The model under review builds one solid part; all positions refer to its coordinate system, in mm. Face numbers are marked on the shaded views. A direction names the side the tool comes from. Give positions to 0.01 mm unless a question says otherwise; leave off trailing zeros. Order: outer loops, then holes, each group sorted by start corner. A loop starts at its lowest first (then second) coordinate and runs counter-clockwise, first axis right, second up. Notation, with made-up numbers: M 69,-24 L 88,-24 A9 cw 88,-9 Z; hole C 11.25,65 d5. An arc over 180 degrees is marked long. One line per question, with ' | ' between items. Start each with the question number.
1. We need section C-C on x = -9.65. Write out the cut boundary in (y, z).
2. For the marked faces 1, 2, 3 and 4, list the 3-axis set-ups (+Z, -Z, +X, -X, +Y, -Y) from which the entire face can be reached by the end or side of a thin tool; tool diameter is ignored.
3. Insertion check: P1, Ø5, axis at y = -5.5, z = 6, coming from the +X side; P2, Ø4.5, axis at y = -6.5, z = 4.5, coming from the -X side; P3, Ø5, axis at x = -35, y = -2.5, coming from the +Z side. Each pin has a flat end and moves straight along its axis. Give the tip position at first contact, or say it passes through.
4. We need section D-D on y = -2.5. Count the separate pieces of the cut face and the enclosed holes in it, then the cut area to 3 significant figures.
5. Wall thickness on L1, parallel to X at y = -0.5, z = 5; L2, parallel to X at y = 1.2, z = 0; L3, parallel to X at y = -7.75, z = -6.75: over which ranges is each line inside the solid? List them lowest first.
6. We need section B-B on x = 24.5. Write out the cut boundary in (y, z), then the cut area to 3 significant figures.
7. We need section A-A on y = -6. Write out the cut boundary in (x, z), then the cut area to 3 significant figures.
```python
from build123d import *

# Parameters (mm, degrees)
SKETCH2_W           = 58
SKETCH2_H           = 20.5
SKETCH2_R           = 8
SKETCH2_R_2         = 1.55
BOSS_EXTRUDE1_DEPTH = 2
SKETCH3_W           = 8.35
SKETCH3_H           = 8.75
SKETCH3_R           = 1.55
BOSS_EXTRUDE2_DEPTH = 9
SKETCH4_W           = 10.5
SKETCH4_H           = 11
SKETCH4_R           = 1.5
BOSS_EXTRUDE3_DEPTH = 2


with BuildPart() as part:
    # Sketch2 → Boss-Extrude1 (new body)
    with BuildSketch(Plane(origin=(0, 0, 0), x_dir=(1, 0, 0), z_dir=(0, 1, 0))):
        Rectangle(SKETCH2_W, SKETCH2_H)
        with Locations((-9.65, 0)):
            Circle(SKETCH2_R, mode=Mode.SUBTRACT)
        with Locations((-24.5, 5)):
            Circle(SKETCH2_R_2, mode=Mode.SUBTRACT)
        with Locations((-24.5, -5)):
            Circle(SKETCH2_R_2, mode=Mode.SUBTRACT)
        with Locations((24.5, 5)):
            Circle(SKETCH2_R_2, mode=Mode.SUBTRACT)
        with Locations((24.5, -5)):
            Circle(SKETCH2_R_2, mode=Mode.SUBTRACT)
        with Locations((9.65, 0)):
            Circle(SKETCH2_R, mode=Mode.SUBTRACT)
    extrude(amount=BOSS_EXTRUDE1_DEPTH)

    # Sketch3 → Boss-Extrude2 (add)
    with BuildSketch(Plane.XZ):
        with Locations((-24.825, 5.875)):
            Rectangle(SKETCH3_W, SKETCH3_H)
        with Locations((-24.5, 5)):
            Circle(SKETCH3_R, mode=Mode.SUBTRACT)
        with Locations((-24.825, -5.875)):
            Rectangle(SKETCH3_W, SKETCH3_H)
        with Locations((-24.5, -5)):
            Circle(SKETCH3_R, mode=Mode.SUBTRACT)
        with Locations((24.825, 5.875)):
            Rectangle(SKETCH3_W, SKETCH3_H)
        with Locations((24.5, 5)):
            Circle(SKETCH3_R, mode=Mode.SUBTRACT)
        with Locations((24.825, -5.875)):
            Rectangle(SKETCH3_W, SKETCH3_H)
        with Locations((24.5, -5)):
            Circle(SKETCH3_R, mode=Mode.SUBTRACT)
    extrude(amount=BOSS_EXTRUDE2_DEPTH)

    # Sketch4 → Boss-Extrude3 (add)
    with BuildSketch(Plane(origin=(0, 0, -10.25), x_dir=(-1, 0, 0), z_dir=(0, 0, -1))):
        with Locations((34.25, -3.5)):
            Rectangle(SKETCH4_W, SKETCH4_H)
        with Locations((35, -2.5)):
            Circle(SKETCH4_R, mode=Mode.SUBTRACT)
        with Locations((-34.25, -3.5)):
            Rectangle(SKETCH4_W, SKETCH4_H)
        with Locations((-35, -2.5)):
            Circle(SKETCH4_R, mode=Mode.SUBTRACT)
    extrude(amount=-BOSS_EXTRUDE3_DEPTH)


solid = part.part
```
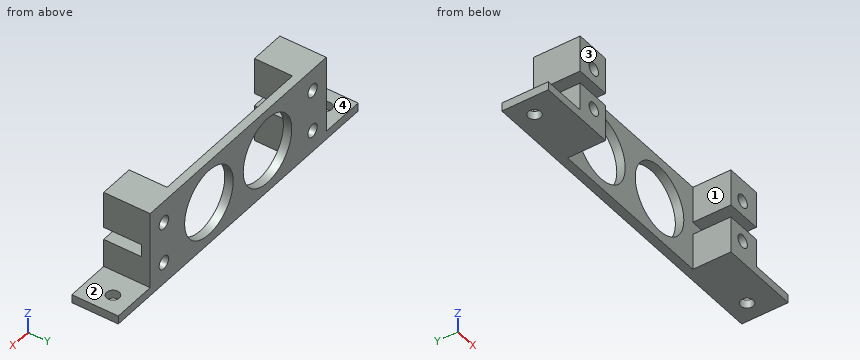
Entries:
1) outline: M 0,-10.25 L 2,-10.25 L 2,-8 L 0,-8 Z; M 0,8 L 2,8 L 2,10.25 L 0,10.25 Z
2) face 1: +Z, -Z, -Y | face 2: +Z, +X, +Y, -Y | face 3: +Z, -Z, +X, -X, -Y | face 4: +Z, -X, +Y, -Y
3) P1: stops at x = 29 | P2: stops at x = -29 | P3: stops at z = -8.25
4) separate pieces: 6 | enclosed holes: 4 | area: 292 mm^2
5) L1: x = -29 to -26.05, -22.95 to -20.65, 20.65 to 22.95, 26.05 to 29 | L2: x = -29 to -17.65, -1.65 to 1.65, 17.65 to 29 | L3: x = -29 to -20.65, 20.65 to 29
6) outline: M -9,-10.25 L 2,-10.25 L 2,-6.55 L -9,-6.55 Z; M -9,-3.45 L 2,-3.45 L 2,3.45 L -9,3.45 L -9,1.5 L 0,1.5 L 0,-1.5 L -9,-1.5 Z; M -9,6.55 L 2,6.55 L 2,10.25 L -9,10.25 Z | area: 130 mm^2
7) outline: M -39.5,-10.25 L -20.65,-10.25 L -20.65,-1.5 L -29,-1.5 L -29,-8.25 L -39.5,-8.25 Z; M -29,1.5 L -20.65,1.5 L -20.65,10.25 L -29,10.25 Z; M 20.65,-10.25 L 39.5,-10.25 L 39.5,-8.25 L 29,-8.25 L 29,-1.5 L 20.65,-1.5 Z; M 20.65,1.5 L 29,1.5 L 29,10.25 L 20.65,10.25 Z; hole C -24.5,-5 d3.1; hole C -24.5,5 d3.1; hole C 24.5,-5 d3.1; hole C 24.5,5 d3.1 | area: 304 mm^2
